Geometry: final body of the model. Coordinates: model frame, mm. A direction names the side the tool comes from. Coordinates: 2 decimals unless noted, no trailing zeros. Write each loop counter-clockwise with the first axis right and the second up, starting at its lowest first coordinate (ties: lowest second). Pieces come first, ordered by that corner, then holes. Notation, with made-up numbers: (62.5, -36) - (113.5, -36) arc R23 cw to (113.5, -25) - close; hole circle Ø4 at (77.25, 32). An arc over 180 degrees is marked (long way). Put each result on its own line as item: value.
```python
from build123d import *

# Parameters (mm, degrees)
SKETCH1_W           = 58
SKETCH1_H           = 44
SKETCH1_W_2         = 56.5
SKETCH1_H_2         = 42.5
BOSS_EXTRUDE1_DEPTH = 10
SKETCH2_W           = 58
SKETCH2_H           = 44
BOSS_EXTRUDE2_DEPTH = 2


with BuildPart() as part:
    # Sketch1 → Boss-Extrude1 (new body)
    with BuildSketch(Plane.XY):
        Rectangle(SKETCH1_W, SKETCH1_H)
        Rectangle(SKETCH1_W_2, SKETCH1_H_2, mode=Mode.SUBTRACT)
    extrude(amount=BOSS_EXTRUDE1_DEPTH)

    # Sketch2 → Boss-Extrude2 (add)
    with BuildSketch(Plane.XY):
        Rectangle(SKETCH2_W, SKETCH2_H)
    extrude(amount=BOSS_EXTRUDE2_DEPTH)


solid = part.part
```
1. Ray query, probe 1 along Y at (x, z) = (-1.5, 7.75); probe 2 along X at (y, z) = (-18.5, 9.5); probe 3 along Z at (x, y) = (11.5, -2). Return the intervals inside material, ascending. Write a range as from..to.
Answer below:
probe 1: y = -22..-21.25, 21.25..22
probe 2: x = -29..-28.25, 28.25..29
probe 3: z = 0..2
2. Section query C-C (x = 7.5). Return loops of the section in (y, z).
Answer below:
outline: (-22, 0) - (22, 0) - (22, 10) - (21.25, 10) - (21.25, 2) - (-21.25, 2) - (-21.25, 10) - (-22, 10) - close
3. Section query B-B (z = 7). Return loops of the section in (x, y), then the cut area to 3 significant figures.
Answer below:
outline: (-29, -22) - (29, -22) - (29, 22) - (-29, 22) - close; hole (-28.25, -21.25) - (28.25, -21.25) - (28.25, 21.25) - (-28.25, 21.25) - close
area: 151 mm²
4. Set-up query: faces 5 (the flat face through (29, 0, 5)), 6 (the flat face through (0, 0, 2)). Return all of +Z, -Z, +X, -X, +Y, -Y with unobstructed straight access to the full face (end or side cutting, diameter ignored); none if empty.
Answer below:
face 5: +Z, -Z, +X, +Y, -Y
face 6: +Z
5. Mould query, pull axis Y, two halves, no side actions, for faces 1 (the flat face through (0, -22, 5)), 2 (the flat face through (0, -21.25, 6)), 3 (the flat face through (-28.25, 0, 6)), 4 (the flat face through (-29, 0, 5)). Classes: +Y half, -Y half, draft (parallel to the pull), parting line (faces both ways), or undercut.
Answer below:
face 1: -Y half
face 2: undercut
face 3: undercut
face 4: draft
6. Pin query (flat end, axial travel): pin 1 Ø10 at (x, y) = (20, 7) entering from +Z; pin 2 Ø1.5 at (x, y) = (1.5, 2) entering from -Z. Return the tip coordinate at first contact, or that it passes through.
Answer below:
pin 1: stops at z = 2
pin 2: stops at z = 0
7. Section query A-A (y = -13). Return loops of the section in (x, z).
Answer below:
outline: (-29, 0) - (29, 0) - (29, 10) - (28.25, 10) - (28.25, 2) - (-28.25, 2) - (-28.25, 10) - (-29, 10) - close
